Part print with two shaded views. Sizes in mm from the minimum x, y, z corner. A direction names the side the tool comes from. Round coordinates to 2 decimals unless told otherwise and drop trailing zeros. Order: outer loops, then holes, each group sorted by start corner. A loop starts at its lowest first (then second) coordinate and runs counter-clockwise, first axis right, second up. Notation, with made-up numbers: (38.5, -1) -> (85.5, -1) arc R24 cw to (85.5, 23) -> close; hole circle Ø9 at (-19, -12.75). An arc over 180 degrees is marked (long way). Put each result on its own line as item: value. Start each with the question number.
Q1. Cut at D-D, the plane y = 30.5. List the corners of the cut face in (x, z), and give its area (3 significant figures).
Q2. Probe L1, parallel to Y at x = 18, z = 10; L2, parallel to Y at x = 116.5, z = 7; L3, parallel to Y at x = 168.5, z = 38.5. List the from-to ranges inside material, lowest first.
Q3. Cut at A-A, the plane z = 22.5. List the corners of the cut face in (x, y), and give its area (3 significant figures).
Q4. Cut at C-C, the plane z = 43. List the corners of the cut face in (x, y).
Q5. Cut at B-B, the plane x = 135. List the corners of the cut face in (y, z), and give its area (3 significant figures).
Q6. 3-axis set-ups, long thin cutter, end or side, ignore diameter. For the marked faces 1 and 2: which of +Z, -Z, +X, -X, +Y, -Y reach the whole face in a straight line?
Q7. Flat gauge pins, fed straight in: P1, Ø5, axis at x = 81.5, z = 28.5, coming from the -Y side; P2, Ø1, axis at x = 41, z = 36, coming from the +Y side; P3, Ø8, axis at x = 46.5, z = 33, coming from the -Y side; P4, Ø2, axis at y = 28.5, z = 37, coming from the +X side. Where does each tip first touch, or does it go through?
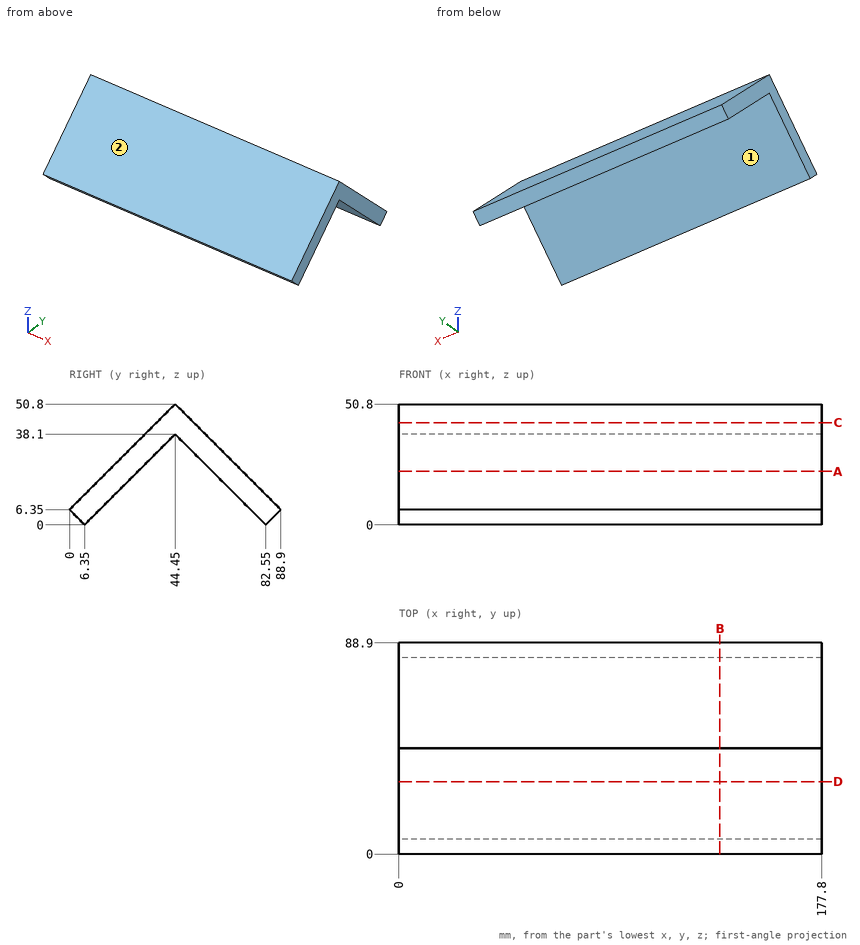
Ans:
1. outline: (0, 24.15) -> (177.8, 24.15) -> (177.8, 36.85) -> (0, 36.85) -> close
1. area: 2,260 mm^2
2. L1: y = 3.65 to 16.35, 72.55 to 85.25
2. L2: y = 0.65 to 13.35, 75.55 to 88.25
2. L3: y = 32.15 to 56.75
3. outline: (0, 16.15) -> (177.8, 16.15) -> (177.8, 28.85) -> (0, 28.85) -> close; (0, 60.05) -> (177.8, 60.05) -> (177.8, 72.75) -> (0, 72.75) -> close
3. area: 4,520 mm^2
4. outline: (0, 36.65) -> (177.8, 36.65) -> (177.8, 52.25) -> (0, 52.25) -> close
5. outline: (0, 6.35) -> (6.35, 0) -> (44.45, 38.1) -> (82.55, 0) -> (88.9, 6.35) -> (44.45, 50.8) -> close
5. area: 1,050 mm^2
6. face 1: -Z, +X, -X
6. face 2: +Z, +X, -X, -Y
7. P1: stops at y = 19.65
7. P2: stops at y = 59.75
7. P3: stops at y = 22.65
7. P4: passes through
